For this review, take the finished solid that the model builds, in its own axes (mm). A direction names the side the tool comes from. Give positions to 0.01 mm unless a question says otherwise; leave off trailing zeros. Write each loop counter-clockwise with the first axis right and the second up, starting at its lowest first coordinate (ties: lowest second). Pieces come first, ordered by that corner, then holes. Notation, with made-up numbers: (0, 66) -> (4, 66) arc R18 cw to (4, 76) -> close; hole circle Ø1 at (17.5, 67.5). An arc over 180 degrees is marked (long way). Answer as CSV lines item,"result".
Autodesk Inventor part; units mm, degrees
ref_plane "YZ Plane" through (0, 0, 0) normal (1, 0, 0) x (0, 1, 0)
ref_plane "XZ Plane" through (0, 0, 0) normal (0, 1, 0) x (-1, 0, 0)
ref_plane "XY Plane" through (0, 0, 0) normal (0, 0, 1) x (1, 0, 0)
sketch "Sketch1" plane through (0, 0, 0) normal (0, 1, 0) x (-1, 0, 0)
  line L0 (0, 0) -> (36, 0)
  line L1 (36, 0) -> (36, -20)
  line L2 (36, -20) -> (0, -20)
  line L3 (0, -20) -> (0, 0)
  dimension "d0" = 36
  dimension "d1" = 20
extrude "Extrusion1" add sketch "Sketch1" along normal blind 2
sketch "Sketch2" plane through (0, 2, 0) normal (0, 1, 0) x (1, 0, 0)
  line L0 (-36, 20) -> (-36, 0)
  line L1 (-36, 10) -> (-32.5, 10)
  circle A0 centre (-32.5, 10) radius 2.6
  point P0 (0, 0)
  dimension "d4" = 3.5
  dimension "d5" = 5.2
extrude "Extrusion2" cut sketch "Sketch2" against normal blind 2
sketch "Sketch3" plane through (-36, 0, 0) normal (0, 0, 1) x (1, 0, 0)
  line L0 (36, 0) -> (0, 0)
  line L1 (0, 0) -> (0, -2)
  line L2 (0, -2) -> (36, 0)
  dimension "d8" = 2
extrude "Extrusion3" add sketch "Sketch3" against normal up to surface (20 mm away)
properties part number "opakowanie"
Q1. Clearance check with flat-ended pins moving along their axes: pin 1 (1.5 mm diameter, centred on x = -14, z = -8.5, fed in from -Y); pin 2 (6 mm diameter, centred on x = -13.5, z = -5.5, fed in from -Y); pin 3 (3 mm diameter, centred on x = -32.5, z = -10, fed in from -Y). State where each tip first meets the part, or that it passes through.
Answer block:
pin 1,"stops at y = -0.82"
pin 2,"stops at y = -0.92"
pin 3,"stops at y = -1.89"
Q2. To check wall thickness, follow probe 1 along X at (y, z) = (1.1, -10); probe 2 along Z at (x, y) = (-32.5, 1.2); probe 3 along X at (y, z) = (0.6, -9). State the ranges of each line that lie inside material, in increasing order. Write a range as [from, to].
Answer block:
probe 1,"x = [-36, -35.1], [-29.9, 0]"
probe 2,"z = [-20, -12.6], [-7.4, 0]"
probe 3,"x = [-36, -34.9], [-30.1, 0]"
Q3. Add section A-A (y = 0.5). Write out the cut boundary in (x, z), plus the area to 3 significant figures.
Answer block:
outline,"(-36, -20) -> (0, -20) -> (0, 0) -> (-36, 0) -> close; hole circle Ø5.2 at (-32.5, -10)"
area,"699 mm2"
Q4. Add section C-C (x = -32.5). Write out the cut boundary in (y, z).
Answer block:
outline,"(-1.81, -20) -> (2, -20) -> (2, -12.6) -> (0, -12.6) -> (0, -7.4) -> (2, -7.4) -> (2, 0) -> (-1.81, 0) -> close"
Q5. Add section D-D (z = -15.75). Write out the cut boundary in (x, y), plus the area to 3 significant figures.
Answer block:
outline,"(-36, -2) -> (0, 0) -> (0, 2) -> (-36, 2) -> close"
area,"108 mm2"
Q6. For faces 1 (the flat face through (-18, 0, -20)), 2 (the cylindrical face through (-34.563, 1.014, -8.418)), list the 3-axis set-ups (+Z, -Z, +X, -X, +Y, -Y) from which the entire face can be reached by the end or side of a thin tool; tool diameter is ignored.
Answer block:
face 1,"-Z, +X, -X, +Y, -Y"
face 2,"+Y"
Q7. Add section B-B (z = -10). Write out the cut boundary in (x, y), plus the area to 3 significant figures.
Answer block:
outline,"(-36, -2) -> (0, 0) -> (0, 2) -> (-29.9, 2) -> (-29.9, 0) -> (-35.1, 0) -> (-35.1, 2) -> (-36, 2) -> close"
area,"97.6 mm2"
Q8. Draft analysis for pull direction X (two halves, no side actions). For faces 3 (the flat face through (-18, -1, -10)), 4 (the flat face through (-18, 0, 0)), 5 (the flat face through (-32, 0, -10)), state which applies: released by +X, released by -X, zero draft, split by the parting line, or undercut.
Answer block:
face 3,"released by +X"
face 4,"zero draft"
face 5,"undercut"
